Check sheet for the drawn part. Datum: minimum x, y, z corner. Units: mm. A direction names the side the tool comes from. Round coordinates to 2 decimals unless told otherwise and drop trailing zeros. Write each loop counter-clockwise with the first axis right and the second up, starting at its lowest first coordinate (ties: lowest second). Pieces come first, ordered by that corner, then holes.
Item 1: Cross-section at A-A on y = 40. Enter the section's corners in (x, z), plus the area to 3 significant figures.
Item 2: Release check for a two-part mould opening along X. For the marked faces 1, 2 and 3 record: +X half, -X half, draft (parallel to the pull), parting line (faces both ways), or undercut.
Item 3: Tool access check on the marked faces 4 and 5. Record the directions out of +Z, -Z, +X, -X, +Y, -Y that give a thin tool (end or side, any length) a straight path to the whole face; none if there is none.
Item 4: Go/stop test with flat-tipped pins: pin 1 Ø3.5 at (x, z) = (5, 3.5) entering from +Y; pin 2 Ø1.8 at (x, z) = (8.5, 4) entering from -Y. Record where each tip stops, or that it passes through.
Item 5: Material ranges on line 1 (X direction, y = 24, z = 0.65); line 2 (X direction, y = 15.5, z = 2.9); line 3 (Y direction, x = 20, z = 1.35), recorded low to high.
Item 6: Cross-section at C-C on y = 18. Enter the section's corners in (x, z), plus the area to 3 significant figures.
Item 7: Cross-section at B-B on x = 20. Enter the section's corners in (y, z).
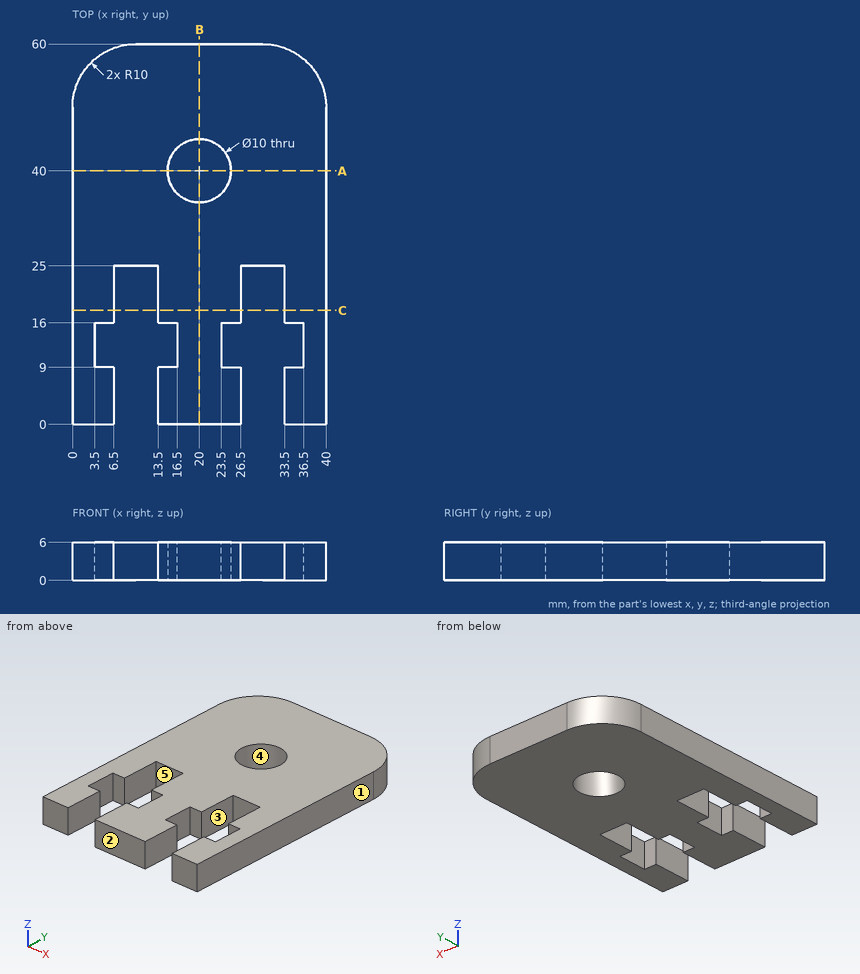
Response values:
1. outline: (0, 0) - (15, 0) - (15, 6) - (0, 6) - close; (25, 0) - (40, 0) - (40, 6) - (25, 6) - close
1. area: 180 mm2
2. face 1: +X half
2. face 2: draft
2. face 3: undercut
3. face 4: +Z, -Z
3. face 5: +Z, -Z, -Y
4. pin 1: stops at y = 59.46
4. pin 2: stops at y = 25
5. line 1: x = 0 to 6.5, 13.5 to 26.5, 33.5 to 40
5. line 2: x = 0 to 3.5, 16.5 to 23.5, 36.5 to 40
5. line 3: y = 0 to 35, 45 to 60
6. outline: (0, 0) - (6.5, 0) - (6.5, 6) - (0, 6) - close; (13.5, 0) - (26.5, 0) - (26.5, 6) - (13.5, 6) - close; (33.5, 0) - (40, 0) - (40, 6) - (33.5, 6) - close
6. area: 156 mm2
7. outline: (0, 0) - (35, 0) - (35, 6) - (0, 6) - close; (45, 0) - (60, 0) - (60, 6) - (45, 6) - close
